Input: dimensioned drawing with shaded views. Units: mm. Origin: part minimum x, y, z. Give positions to 0.01 mm unless a question says otherwise; leave off trailing zeros. Write each loop counter-clockwise with the first axis right and the second up, starting at its lowest first coordinate (ties: lowest second). Pieces come first, ordered by that corner, then holes.
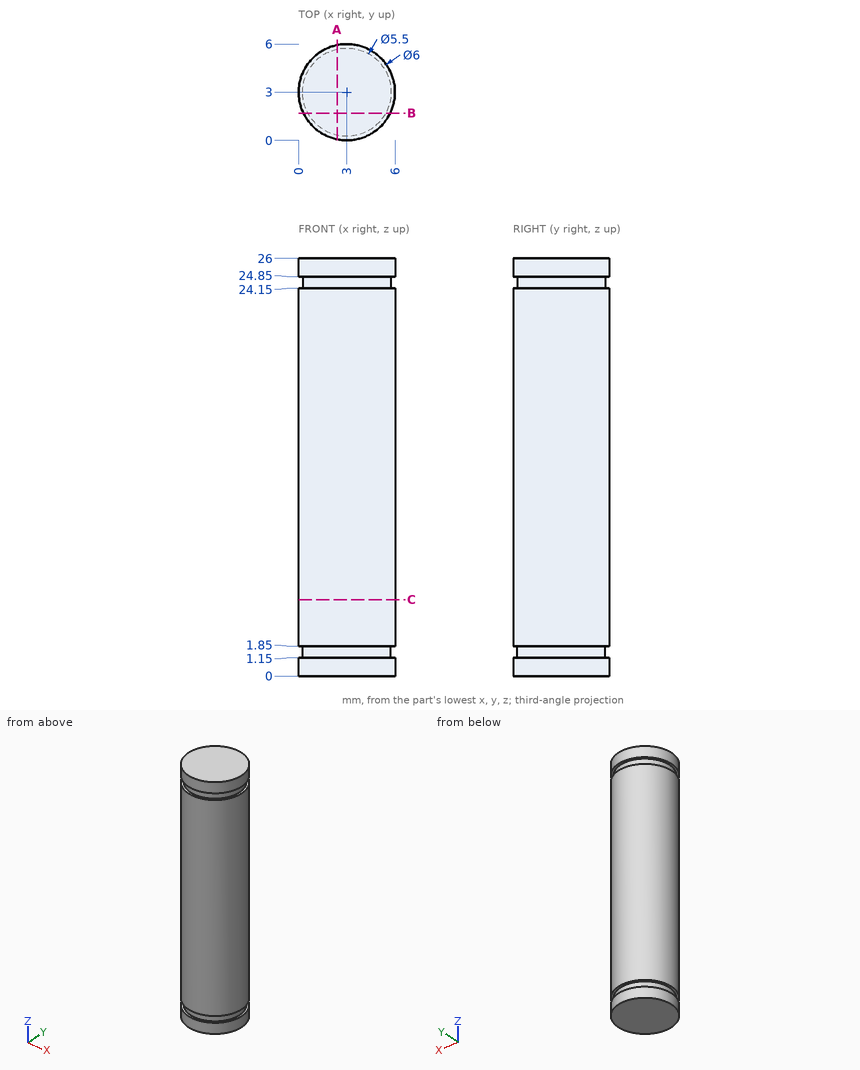
Item 1: Section A-A, the plane x = 2.4. Return the cut outline in (y, z).
Found:
outline: (0.06, 0) - (5.94, 0) - (5.94, 1.15) - (5.68, 1.15) - (5.68, 1.85) - (5.94, 1.85) - (5.94, 24.15) - (5.68, 24.15) - (5.68, 24.85) - (5.94, 24.85) - (5.94, 26) - (0.06, 26) - (0.06, 24.85) - (0.32, 24.85) - (0.32, 24.15) - (0.06, 24.15) - (0.06, 1.85) - (0.32, 1.85) - (0.32, 1.15) - (0.06, 1.15) - close
Item 2: Pin query (flat end, axial travel): pin 1 Ø1 at (y, z) = (2, 20.5) entering from -X; pin 2 Ø1.5 at (x, z) = (1.5, 5.5) entering from +Y. Return the tip coordinate at first contact, or that it passes through.
Found:
pin 1: stops at x = 0.04
pin 2: stops at y = 5.9
Item 3: Line query: L1, parallel to Z at x = 5.6, y = 4; L2, parallel to X at y = 2.9, z = 17.75; L3, parallel to X at y = 0.35, z = 5.5. Output: solid intervals per line, ascending.
Found:
L1: z = 0 to 1.15, 1.85 to 24.15, 24.85 to 26
L2: x = 0 to 6
L3: x = 1.59 to 4.41
Item 4: Section C-C, the plane z = 4.75. Return the cut outline in (x, y).
Found:
outline: circle Ø6 at (3, 3)
Item 5: Section B-B, the plane y = 1.7. Return the cut outline in (x, z).
Found:
outline: (0.3, 0) - (5.7, 0) - (5.7, 1.15) - (5.42, 1.15) - (5.42, 1.85) - (5.7, 1.85) - (5.7, 24.15) - (5.42, 24.15) - (5.42, 24.85) - (5.7, 24.85) - (5.7, 26) - (0.3, 26) - (0.3, 24.85) - (0.58, 24.85) - (0.58, 24.15) - (0.3, 24.15) - (0.3, 1.85) - (0.58, 1.85) - (0.58, 1.15) - (0.3, 1.15) - close
